Source: CAD feature listing. Evaluate the final solid. Frame: model axes, mm. A direction names the side the tool comes from. Give positions to 0.01 mm unless a question says otherwise; leave off trailing zeros. Loops run counter-clockwise (first coordinate to the right, second up) from the corner with the lowest first, then second, coordinate; pieces in that order, holes last. Notation, with made-up numbers: (73, 13.25) - (108, 13.25) arc R26 cw to (108, 51.25) - close; hole circle Ø2 at (88.5, 32). An arc over 180 degrees is marked (long way). Write each question's results on one line, items separated by ' | '. Start each with the question number.
(1) Cut plane A-A on z = -2.5. Return the cut outline in (x, y), then the cut area to 3 significant figures.
(2) Cut plane C-C on z = 10. Return the cut outline in (x, y), then the cut area to 3 significant figures.
(3) Reachability of faces 5 (the cylindrical face through (-14.248, 1.521, 14.287)), 6 (the cylindrical face through (-45.07, 2.01, -9.18)), 7 (the flat face through (59.5, 1, 0)) from +Z, -Z, +X, -X, +Y, -Y: full face, straight path, thin tool, end or side. Return the list, or none.
(4) Cut plane B-B on x = 49.5. Return the cut outline in (y, z).
(5) Pull-direction query (Z, two-part tool) for faces 1 (the flat face through (-1, 0, -20)), 2 (the flat face through (-1, 1, -22)), 3 (the flat face through (0, 2, -15)), 4 (the flat face through (15, 2, 0)); classes: pulls with the +Z half, pulls with the -Z half, needs draft (parallel to the pull), parting line crosses it, or undercut.
(6) Cut plane D-D on z = -9.5. Return the cut outline in (x, y), then the cut area to 3 significant figures.
(7) Material intervals for line 1 along X through (y, z) = (2.45, 12); line 2 along Z through (x, y) = (49.5, 2); line 3 along Z through (x, y) = (12, 1.2), sorted ascending. Write a range as [from, to].
(8) Contact query for a flat-ended pin moving along its axis: pin 1 (6.5 mm diameter, centred on x = 49.5, z = -12, fed in from +Y). Output: stop coordinate, or through.
from build123d import *

# Parameters (mm, degrees)
ESBO_O1_W                 = 119
ESBO_O1_H                 = 44
EXTRUS_O1_DEPTH           = 3
ESBO_O2_R                 = 5.25
EXTRUS_O2_DEPTH           = 2
ESPELHAR2_COPY_1_SKETCH_R = 5.25
ESPELHAR2_COPY_1_DEPTH    = 2
EXTRUS_O3_DEPTH           = 3


with BuildPart() as part:
    # Esboço1 → Extrusão1 (new body)
    with BuildSketch(Plane(origin=(0, 0, 0), x_dir=(1, 0, 0), z_dir=(0, 1, 0))):
        Rectangle(ESBO_O1_W, ESBO_O1_H)
    extrude(amount=EXTRUS_O1_DEPTH)

    # Esboço2 → Extrusão2 (cut)
    with BuildSketch(Plane(origin=(0, 3, 0), x_dir=(1, 0, 0), z_dir=(0, 1, 0))):
        with Locations(Location((-49.5, 12, 0), (0, 0, 270))):
            Circle(ESBO_O2_R)
    extrus_o2 = extrude(amount=-EXTRUS_O2_DEPTH, mode=Mode.SUBTRACT)

    # Espelhar1: Extrusão2 across plane
    add(extrus_o2.mirror(Plane(origin=(0, 0, 0), x_dir=(0, 0, 1), z_dir=(1, 0, 0))), mode=Mode.SUBTRACT)

    # Espelhar2: Extrusão2 across plane
    add(extrus_o2.mirror(Plane.XY), mode=Mode.SUBTRACT)

    # Espelhar2 copy 1 sketch → Espelhar2 copy 1 (cut)
    with BuildSketch(Plane(origin=(0, 3, 0), x_dir=(-1, 0, 0), z_dir=(0, 1, 0))):
        with Locations(Location((-49.5, 12, 0), (0, 0, 270))):
            Circle(ESPELHAR2_COPY_1_SKETCH_R)
    extrude(amount=-ESPELHAR2_COPY_1_DEPTH, mode=Mode.SUBTRACT)

    # Esboço3 → Extrusão3 (cut)
    with BuildSketch(Plane(origin=(0, 3, 0), x_dir=(1, 0, 0), z_dir=(0, 1, 0))):
        with BuildLine():
            Line((-12.5, 15), (12.5, 15))
            ThreePointArc((12.5, 15), (14.267766953, 14.267766953), (15, 12.5))
            Line((15, 12.5), (15, -12.5))
            ThreePointArc((15, -12.5), (14.267766953, -14.267766953), (12.5, -15))
            Line((12.5, -15), (-12.5, -15))
            ThreePointArc((-12.5, -15), (-14.267766953, -14.267766953), (-15, -12.5))
            Line((-15, -12.5), (-15, 12.5))
            ThreePointArc((-15, 12.5), (-14.267766953, 14.267766953), (-12.5, 15))
        make_face()
    extrude(amount=-EXTRUS_O3_DEPTH, mode=Mode.SUBTRACT)


solid = part.part
Ans:
1) outline: (-59.5, 0) - (-15, 0) - (-15, 3) - (-59.5, 3) - close; (15, 0) - (59.5, 0) - (59.5, 3) - (15, 3) - close | area: 267 mm^2
2) outline: (-59.5, 0) - (-15, 0) - (-15, 3) - (-44.65, 3) - (-44.65, 1) - (-54.35, 1) - (-54.35, 3) - (-59.5, 3) - close; (15, 0) - (59.5, 0) - (59.5, 3) - (54.35, 3) - (54.35, 1) - (44.65, 1) - (44.65, 3) - (15, 3) - close | area: 228 mm^2
3) face 5: +Y, -Y | face 6: +Y | face 7: +Z, -Z, +X, +Y, -Y
4) outline: (0, -22) - (3, -22) - (3, -17.25) - (1, -17.25) - (1, -6.75) - (3, -6.75) - (3, 6.75) - (1, 6.75) - (1, 17.25) - (3, 17.25) - (3, 22) - (0, 22) - close
5) face 1: needs draft | face 2: pulls with the -Z half | face 3: undercut | face 4: undercut
6) outline: (-59.5, 0) - (-15, 0) - (-15, 3) - (-44.88, 3) - (-44.88, 1) - (-54.12, 1) - (-54.12, 3) - (-59.5, 3) - close; (15, 0) - (59.5, 0) - (59.5, 3) - (54.12, 3) - (54.12, 1) - (44.88, 1) - (44.88, 3) - (15, 3) - close | area: 230 mm^2
7) line 1: [-59.5, -54.75], [-44.25, -15], [15, 44.25], [54.75, 59.5] | line 2: [-22, -17.25], [-6.75, 6.75], [17.25, 22] | line 3: [-22, -15], [15, 22]
8) pin 1: y = 1
